from build123d import *

# Parameters (mm, degrees)
F0_W     = 168.208927
F0_H     = 50.145343
F1_DEPTH = 25
F2_W     = 164.286842
F2_H     = 45.602561
F3_DEPTH = 21
F4_W     = 2.237212
F4_H     = 45.602561
F4_W_2   = 2.23721
F4_W_3   = 2.259579
F4_W_4   = 2.25958
F4_W_5   = 1.535502
F4_W_6   = 2.804493
F5_DEPTH = 2.4


with BuildPart() as f1:
    # F0 (on Top) → F1 (new body)
    with BuildSketch(Plane.XY):
        with Locations((18.128507, -7.140766)):
            Rectangle(F0_W, F0_H)
    extrude(amount=F1_DEPTH)

    # F2 (on face) → F3 (cut)
    with BuildSketch(Plane.XY.offset(25)):
        with Locations((18.128509, -7.140767)):
            Rectangle(F2_W, F2_H)
    extrude(amount=-F3_DEPTH, mode=Mode.SUBTRACT)

    # F4 (on face) → F5 (join)
    with BuildSketch(Plane.XY.offset(4)):
        with Locations((-53.010842, -7.140767)):
            Rectangle(F4_W, F4_H)
        with Locations((-40.482435, -7.140767)):
            Rectangle(F4_W_2, F4_H)
        with Locations((-27.954025, -7.140767)):
            Rectangle(F4_W_2, F4_H)
        with Locations((-17.662825, -7.140767)):
            Rectangle(F4_W_2, F4_H)
        with Locations((-5.134415, -7.140767)):
            Rectangle(F4_W_2, F4_H)
        with Locations((7.393995, -7.140767)):
            Rectangle(F4_W_2, F4_H)
        with Locations((-46.746636, -7.140767)):
            Rectangle(F4_W_3, F4_H)
        with Locations((-34.21823, -7.140767)):
            Rectangle(F4_W_4, F4_H)
        with Locations((-23.564991, -7.140767)):
            Rectangle(F4_W_5, F4_H)
        with Locations((-11.39862, -7.140767)):
            Rectangle(F4_W_4, F4_H)
        with Locations((1.402246, -7.140767)):
            Rectangle(F4_W_6, F4_H)
        with Locations((13.647015, -7.140767)):
            Rectangle(F4_W_2, F4_H)
    extrude(amount=F5_DEPTH)


solid = f1.part
For this review, take the finished solid that the model builds, in its own axes (mm). A direction names the side the tool comes from. Give positions to 0.01 mm unless a question says otherwise; leave off trailing zeros. Order: outer loops, then holes, each group sorted by start corner. A loop starts at its lowest first (then second) coordinate and runs counter-clockwise, first axis right, second up. Notation, with made-up numbers: (16.5, 60.25) - (47.5, 60.25) arc R37 cw to (47.5, 97.25) - close; hole circle Ø1 at (61, 26.25). An arc over 180 degrees is marked (long way). Answer as a JSON object with one key per item and string values. Group by question number.
Item 1: Draft analysis for pull direction Y (two halves, no side actions). For faces 1 (the flat face through (-44, -7, 4)), 2 (the flat face through (17, 17.932, 12)), 3 (the flat face through (17, -32.213, 12)), 4 (the flat face through (-65.976, -7, 12)), state which applies: pulls with the +Y half, pulls with the -Y half, needs draft (parallel to the pull), parting line crosses it, or undercut.
Item 2: Take a section at A-A on z = 14.25. Give the boundary of the cut face in (x, y).
Item 3: Machinability: for faces 5 (the flat face through (102.233, -7, 12)), 6 (the flat face through (-8, -7, 4)), which of the approach directions +Z, -Z, +X, -X, +Y, -Y give a long, thin tool a straight path to every point of the face, cutting with its end or side? Answer none if there is none.
Item 4: Clearance check with flat-ended pins moving along their axes: pin 1 Ø1.2 at (x, y) = (-8.5, -5) entering from +Z; pin 2 Ø3 at (x, y) = (1, -3) entering from +Z. State where each tip first meets the part, or that it passes through.
Item 5: Wall thickness on line 1 along Y through (x, z) = (48, 24.25); line 2 along X through (y, z) = (-15.5, 19.5); line 3 along Z through (x, y) = (12, -17.5): over which ranges is each line inside the solid? List them lowest first.
Item 6: Take a section at B-B on x = 66. Give the boundary of the cut face in (y, z), and give its area (3 significant figures).
Reported:
{
 "1": {"face 1": "undercut", "face 2": "pulls with the +Y half", "face 3": "pulls with the -Y half", "face 4": "needs draft"},
 "2": {"outline": "(-65.98, -32.21) - (102.23, -32.21) - (102.23, 17.93) - (-65.98, 17.93) - close; hole (-64.01, -29.94) - (100.27, -29.94) - (100.27, 15.66) - (-64.01, 15.66) - close"},
 "3": {"face 5": "+Z, -Z, +X, +Y, -Y", "face 6": "+Z"},
 "4": {"pin 1": "z = 4", "pin 2": "z = 6.4"},
 "5": {"line 1": "-32.21 to -29.94, 15.66 to 17.93", "line 2": "-65.98 to -64.01, 100.27 to 102.23", "line 3": "0 to 4"},
 "6": {"outline": "(-32.21, 0) - (17.93, 0) - (17.93, 25) - (15.66, 25) - (15.66, 4) - (-29.94, 4) - (-29.94, 25) - (-32.21, 25) - close", "area": "296 mm^2"}
}
